Check sheet for the modelled part. Datum: model origin and axes. Units: mm. Face numbers are marked on the shaded views. A direction names the side the tool comes from. Coordinates: 2 decimals unless noted, no trailing zeros. Write each loop counter-clockwise with the first axis right and the second up, starting at its lowest first coordinate (ties: lowest second). Pieces come first, ordered by that corner, then holes. Notation, with made-up numbers: (57.5, 4) -> (91.5, 4) arc R7 ccw to (91.5, 16) -> close; hole circle Ø11 at (64, -13.75). An arc over 180 degrees is marked (long way). Put each result on its own line as item: value.
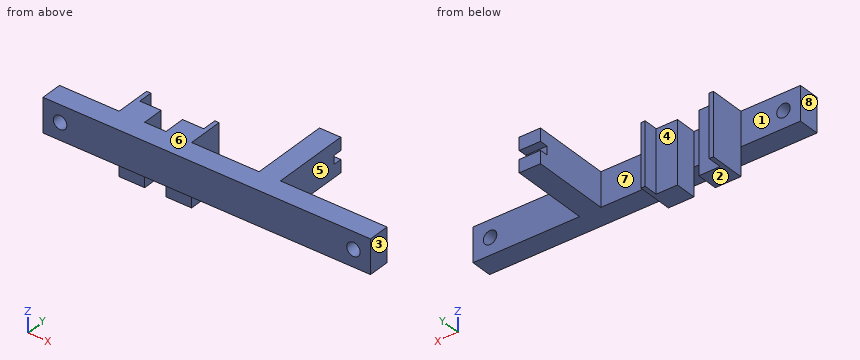
```python
from build123d import *

# Parameters (mm, degrees)
SKETCH1_W           = 230.5
SKETCH1_H           = 24
BOSS_EXTRUDE1_DEPTH = 15
SKETCH2_R           = 4.75
CUT_EXTRUDE1_DEPTH  = 15
SKETCH4_W           = 18
SKETCH4_H           = 44
BOSS_EXTRUDE2_DEPTH = 15
SKETCH5_W           = 15
SKETCH5_H           = 24
BOSS_EXTRUDE3_DEPTH = 49
SKETCH6_W           = 15
SKETCH6_H           = 9
BOSS_EXTRUDE4_DEPTH = 6
SKETCH7_W           = 3
SKETCH7_H           = 44
BOSS_EXTRUDE5_DEPTH = 10


with BuildPart() as part:
    # Sketch1 → Boss-Extrude1 (new body)
    with BuildSketch(Plane(origin=(0, 0, 0), x_dir=(1, 0, 0), z_dir=(0, 1, 0))):
        with Locations((21.518565941, 35.196222791)):
            Rectangle(SKETCH1_W, SKETCH1_H)
    extrude(amount=BOSS_EXTRUDE1_DEPTH)

    # Sketch2 → Cut-Extrude1 (cut)
    with BuildSketch(Plane(origin=(0, 15, 0), x_dir=(1, 0, 0), z_dir=(0, 1, 0))):
        with Locations(Location((-81.731434059, 35.196222791, 0), (0, 0, 270))):
            Circle(SKETCH2_R)
        with Locations(Location((124.768565941, 35.196222791, 0), (0, 0, 270))):
            Circle(SKETCH2_R)
    extrude(amount=-CUT_EXTRUDE1_DEPTH, mode=Mode.SUBTRACT)

    # Sketch4 → Boss-Extrude2 (add)
    with BuildSketch(Plane(origin=(0, 15, 0), x_dir=(1, 0, 0), z_dir=(0, 1, 0))):
        with Locations((-42.731434059, 45.196222791)):
            Rectangle(SKETCH4_W, SKETCH4_H)
        with Locations((-9.731434059, 45.196222791)):
            Rectangle(SKETCH4_W, SKETCH4_H)
    extrude(amount=BOSS_EXTRUDE2_DEPTH)

    # Sketch5 → Boss-Extrude3 (add)
    with BuildSketch(Plane(origin=(0, 15, 0), x_dir=(1, 0, 0), z_dir=(0, 1, 0))):
        with Locations((54.268565941, 35.196222791)):
            Rectangle(SKETCH5_W, SKETCH5_H)
    extrude(amount=BOSS_EXTRUDE3_DEPTH)

    # Sketch6 → Boss-Extrude4 (add)
    with BuildSketch(Plane(origin=(0, 64, 0), x_dir=(1, 0, 0), z_dir=(0, 1, 0))):
        with Locations((54.268565941, 42.696222791)):
            Rectangle(SKETCH6_W, SKETCH6_H)
        with Locations((54.268565941, 27.696222791)):
            Rectangle(SKETCH6_W, SKETCH6_H)
    extrude(amount=BOSS_EXTRUDE4_DEPTH)

    # Sketch7 → Boss-Extrude5 (add)
    with BuildSketch(Plane(origin=(0, 30, 0), x_dir=(1, 0, 0), z_dir=(0, 1, 0))):
        with Locations((-50.231434059, 45.196222791)):
            Rectangle(SKETCH7_W, SKETCH7_H)
        with Locations((-2.231434059, 45.196222791)):
            Rectangle(SKETCH7_W, SKETCH7_H)
    extrude(amount=BOSS_EXTRUDE5_DEPTH)


solid = part.part
```
Q1. Cross-section at C-C (y = 35.5). Record the cut outline in (x, z), plus the area to 3 significant figures.
Recorded:
outline: (-51.73, -67.2) -> (-48.73, -67.2) -> (-48.73, -23.2) -> (-51.73, -23.2) -> close; (-3.73, -67.2) -> (-0.73, -67.2) -> (-0.73, -23.2) -> (-3.73, -23.2) -> close; (46.77, -47.2) -> (61.77, -47.2) -> (61.77, -23.2) -> (46.77, -23.2) -> close
area: 624 mm2
Q2. Cross-section at D-D (y = 6). Record the cut outline in (x, z).
Recorded:
outline: (-93.73, -47.2) -> (136.77, -47.2) -> (136.77, -23.2) -> (-93.73, -23.2) -> close; hole circle Ø9.5 at (-81.73, -35.2); hole circle Ø9.5 at (124.77, -35.2)
Q3. Tool access check on the marked faces 1, 2, 3, 4 and 5. Record the directions out of +Z, -Z, +X, -X, +Y, -Y that give a thin tool (end or side, any length) a straight path to the whole face; none if there is none.
Recorded:
face 1: +Z, -Z, -X, +Y
face 2: -Z, +X, -X, +Y, -Y
face 3: +Z, -Z, +X, +Y, -Y
face 4: +Z, -Z, +Y
face 5: +Z, -Z, +X, +Y
Q4. Cross-section at A-A (y = 22). Record the cut outline in (x, z), plus the area to 3 significant figures.
Recorded:
outline: (-51.73, -67.2) -> (-33.73, -67.2) -> (-33.73, -23.2) -> (-51.73, -23.2) -> close; (-18.73, -67.2) -> (-0.73, -67.2) -> (-0.73, -23.2) -> (-18.73, -23.2) -> close; (46.77, -47.2) -> (61.77, -47.2) -> (61.77, -23.2) -> (46.77, -23.2) -> close
area: 1,940 mm2
Q5. Material ranges on line 1 along X through (y, z) = (37.5, -33.5); line 2 along X through (y, z) = (31, -50.5); line 3 along X through (y, z) = (16, -53.5), recorded low to high.
Recorded:
line 1: x = -51.73 to -48.73, -3.73 to -0.73, 46.77 to 61.77
line 2: x = -51.73 to -48.73, -3.73 to -0.73
line 3: x = -51.73 to -33.73, -18.73 to -0.73
Q6. Mould release check, pull along X, two halves, no side actions. Record for the marked faces 6, 7 and 8: released by +X, released by -X, zero draft, split by the parting line, or undercut.
Recorded:
face 6: zero draft
face 7: undercut
face 8: released by -X
Q7. Cross-section at B-B (z = -49.5). Record the cut outline in (x, y), plus the area to 3 significant figures.
Recorded:
outline: (-51.73, 15) -> (-33.73, 15) -> (-33.73, 30) -> (-48.73, 30) -> (-48.73, 40) -> (-51.73, 40) -> close; (-18.73, 15) -> (-0.73, 15) -> (-0.73, 40) -> (-3.73, 40) -> (-3.73, 30) -> (-18.73, 30) -> close
area: 600 mm2
Q8. Depth check by flat-ended pin: P1, Ø10, axis at x = 65.5, z = -53, coming from the -Y side; P2, Ø4, axis at y = 18, z = -41.5, coming from the +X side; P3, Ø1.5, axis at x = -51, z = -40.5, coming from the +Y side; P4, Ø9, axis at x = -10.5, z = -61, coming from the -Y side. Enter the tip coordinate at first touch or a pass-through.
Recorded:
P1: passes through
P2: stops at x = 61.77
P3: stops at y = 40
P4: stops at y = 15
